from build123d import *

# Parameters (mm, degrees)
F0_R      = 8.6637425689
F1_DEPTH  = 25.4
F3_DEPTH  = 12.7
F4_R      = 5.08
F5_R      = 5.08
F6_R      = 12.7
F7_R      = 12.69999
F8_R      = 12.7
F9_R      = 12.69999
F10_R     = 5.5257991494
F11_DEPTH = 25.4
F12_R     = 5.5331253453
F13_DEPTH = 25.4


# Not quite as in the source:
# - a fillet or chamfer is up to 0.001 mm smaller than in the source, because OpenCascade refuses the exact size


with BuildPart() as f1:
    # F0 (on Top) → F1 (new body)
    with BuildSketch(Plane.XY):
        with BuildLine():
            ThreePointArc((19.1970299929, 44.4350838661), (0, 63.6321138591), (-19.1970299929, 44.4350838661))
            Line((-19.1970299929, 44.4350838661), (-19.1970299929, -44.4350838661))
            ThreePointArc((-19.1970299929, -44.4350838661), (0, -63.6321138591), (19.1970299929, -44.4350838661))
            Line((19.1970299929, -44.4350838661), (19.1970299929, 44.4350838661))
        make_face()
        with Locations((0, -44.4350838661)):
            Circle(F0_R, mode=Mode.SUBTRACT)
        with Locations((0, 44.4350838661)):
            Circle(F0_R, mode=Mode.SUBTRACT)
    extrude(amount=-F1_DEPTH)

    # F2 (on Right) → F3 (join, symmetric)
    with BuildSketch(Plane.YZ):
        Polygon((-32.3530361056, 35.0379385054), (-32.3530361056, 0), (31.0105849057, 0), (31.0105849057, 35.0379385054), (17.0491095632, 35.0379385054), (17.0491095632, 9.5313927159), (-18.3915607631, 9.5313927159), (-18.3915607631, 35.0379385054), align=None)
    extrude(amount=F3_DEPTH, both=True)

    # F4
    f4_edges = [f1.edges().sort_by_distance(p)[0] for p in [
        (0, -18.391561, 9.531393),
    ]]
    fillet(f4_edges, radius=F4_R)

    # F5
    f5_edges = [f1.edges().sort_by_distance(p)[0] for p in [
        (0, 17.04911, 9.531393),
    ]]
    fillet(f5_edges, radius=F5_R)

    # F6
    f6_edges = [f1.edges().sort_by_distance(p)[0] for p in [
        (12.7, -25.372298, 35.037939),
    ]]
    fillet(f6_edges, radius=F6_R)

    # F7 (radius 12.7 in the source; OpenCascade refuses exactly that, so slightly less here)
    f7_edges = [f1.edges().sort_by_distance(p)[0] for p in [
        (-12.7, -25.372298, 35.037939),
    ]]
    fillet(f7_edges, radius=F7_R)

    # F8
    f8_edges = [f1.edges().sort_by_distance(p)[0] for p in [
        (12.7, 24.029847, 35.037939),
    ]]
    fillet(f8_edges, radius=F8_R)

    # F9 (radius 12.7 in the source; OpenCascade refuses exactly that, so slightly less here)
    f9_edges = [f1.edges().sort_by_distance(p)[0] for p in [
        (-12.7, 24.029847, 35.037939),
    ]]
    fillet(f9_edges, radius=F9_R)

    # F10 (on face) → F11 (cut)
    with BuildSketch(Plane(origin=(0, 31.0105849057, 0), x_dir=(-1, 0, 0), z_dir=(0, 1, 0))):
        with Locations((0, 22.3379385054)):
            Circle(F10_R)
    extrude(amount=-F11_DEPTH, mode=Mode.SUBTRACT)

    # F12 (on face) → F13 (cut)
    with BuildSketch(Plane.XZ.offset(32.3530361056)):
        with Locations((0, 22.3379385054)):
            Circle(F12_R)
    extrude(amount=-F13_DEPTH, mode=Mode.SUBTRACT)


solid = f1.part
Verification items for the finished model (mm, model axes). A direction names the side the tool comes from. Give positions to 0.01 mm unless a question says otherwise; leave off trailing zeros. Write each loop counter-clockwise with the first axis right and the second up, starting at its lowest first coordinate (ties: lowest second). Pieces come first, ordered by that corner, then holes. Notation, with made-up numbers: M 29.25,49 L 69.25,49 A19 ccw 69.25,73 Z; hole C 47.5,-19 d7. An arc over 180 degrees is marked long. Put each result on its own line as item: value. Start each with the question number.
1. Draft check along X on faces 1 (the face through (2.975, -25.47, 27.003)), 2 (the face through (0, 0, 9.531)), 3 (the face through (9.08, 23.93, 31.22)), 4 (the face through (-0.422, -63.627, -12.522)). Enter one of: +X half, -X half, draft (parallel to the pull), parting line (faces both ways), or undercut.
2. Go/stop test with flat-tipped pins: pin 1 Ø20.5 at (x, z) = (5.5, 21) entering from -Y; pin 2 Ø7.5 at (x, z) = (-1.5, 11) entering from +Y; pin 3 Ø7.5 at (x, y) = (1.5, -3) entering from +Z. Record where each tip stops, or that it passes through.
3. Set-up check for faces 5 (the face through (0.18, 15.52, 10.98)), 6 (the face through (12.7, -1, 9)), 7 (the face through (0, 31.011, 13)), 8 (the face through (0, -32.353, 14)), 9 (the face through (-19.197, 1, -13)): record each of +Z, -Z, +X, -X, +Y, -Y from which the full face is reachable in a straight line by a thin tool's end or side.
4. Section check D-D (y = 46). Record the cut outline in (x, z).
5. Section check C-C (x = 4). Give the number of separate pieces and of enclosed holes in the cut face, and give its area (3 significant figures).
6. Scan lines: line 1 along Y through (x, z) = (0, -15); line 2 along Y through (x, z) = (-6, 32.5); line 3 along Y through (x, z) = (-4.5, -7). Record each from-to range of solid material in increasing order. Write a range as [from, to].
7. Section check A-A (z = -15). Record the cut outline in (x, y), and give its area (3 significant figures).
Answer list:
1. face 1: undercut
1. face 2: draft
1. face 3: +X half
1. face 4: parting line
2. pin 1: y = -32.35
2. pin 2: y = 31.01
2. pin 3: z = 9.53
3. face 5: +Z, +X, -X
3. face 6: +Z, +X, +Y, -Y
3. face 7: +Z, +X, -X, +Y
3. face 8: +Z, +X, -X, -Y
3. face 9: +Z, -Z, -X, +Y, -Y
4. outline: M -19.13,-25.4 L -8.52,-25.4 L -8.52,0 L -19.13,0 Z; M 8.52,-25.4 L 19.13,-25.4 L 19.13,0 L 8.52,0 Z
5. separate pieces: 5
5. enclosed holes: 0
5. area: 3,530 mm2
6. line 1: [-63.63, -53.1], [-35.77, 35.77], [53.1, 63.63]
6. line 2: [-32.35, -18.39], [17.05, 31.01]
6. line 3: [-63.1, -51.84], [-37.03, 37.03], [51.84, 63.1]
7. outline: M -19.2,-44.44 A19.2 ccw 19.2,-44.44 L 19.2,44.44 A19.2 ccw -19.2,44.44 Z; hole C 0,-44.44 d17.33; hole C 0,44.44 d17.33
7. area: 4,100 mm2
